CAD build for the part. Positions are in the model's coordinates, mm. A direction names the side the tool comes from. Round coordinates to 2 decimals unless told otherwise and drop trailing zeros. Loops run counter-clockwise (first coordinate to the right, second up) from the corner with the lowest first, then second, coordinate; pieces in that order, holes last.
```python
from build123d import *

# Parameters (mm, degrees)
SKETCH_1_R          = 4
EXTRUDE_1_DEPTH     = 1.5
SKETCH_2_R          = 2.9
EXTRUDE_2_DEPTH     = 5
CUT_EXTRUDE_1_REACH = 10.617
SKETCH_3_R          = 1.6


with BuildPart() as part:
    # 草图1 → 凸台-拉伸1 (new body)
    with BuildSketch(Plane(origin=(0, 0, 0), x_dir=(1, 0, 0), z_dir=(0, 1, 0))):
        with Locations(Location((0, 0, 0), (0, 0, 270))):
            Circle(SKETCH_1_R)
    extrude(amount=EXTRUDE_1_DEPTH)

    # 草图2 → 凸台-拉伸2 (add)
    with BuildSketch(Plane(origin=(0, 1.5, 0), x_dir=(1, 0, 0), z_dir=(0, 1, 0))):
        with Locations(Location((0, 0, 0), (0, 0, 270))):
            Circle(SKETCH_2_R)
    extrude(amount=EXTRUDE_2_DEPTH)

    # 草图3 → 切除-拉伸1 (cut, up to next)
    with BuildSketch(Plane(origin=(0, 6.5, 0), x_dir=(1, 0, 0), z_dir=(0, 1, 0)), mode=Mode.PRIVATE) as cut_extrude_1_sk1:
        with Locations(Location((0, 0, 0), (0, 0, 270))):
            Circle(SKETCH_3_R)
    cut_extrude_1_tool1 = extrude(cut_extrude_1_sk1.sketch, amount=-CUT_EXTRUDE_1_REACH, mode=Mode.PRIVATE) & part.part
    add(cut_extrude_1_tool1.solids().sort_by_distance((0, 6.5, 0))[0], mode=Mode.SUBTRACT)


solid = part.part
```
Item 1: Cut at A-A, the plane x = 0. Give the cut face in (y, z).
Answers follow:
outline: (0, -4) - (1.5, -4) - (1.5, -2.9) - (6.5, -2.9) - (6.5, -1.6) - (0, -1.6) - close; (0, 1.6) - (6.5, 1.6) - (6.5, 2.9) - (1.5, 2.9) - (1.5, 4) - (0, 4) - close
Item 2: Flat gauge pins, fed straight in: P1, Ø1.5, axis at x = 0.5, z = -1.5, coming from the -Y side; P2, Ø1, axis at y = 4, z = -2, coming from the -X side. Where does each tip first touch, or does it go through?
Answers follow:
P1: stops at y = 0
P2: stops at x = -2.48
Item 3: Cut at C-C, the plane y = 2.5. Give the cut face in (x, z).
Answers follow:
outline: circle Ø5.8 at (0, 0); hole circle Ø3.2 at (0, 0)
Item 4: 3-axis set-ups, long thin cutter, end or side, ignore diameter. For faces 1 (the flat face through (-1.25, 6.5, 1.25)), 2 (the cylindrical face through (0.1, 4, -2.9)): which of +Z, -Z, +X, -X, +Y, -Y reach the whole face in a straight line?
Answers follow:
face 1: +Z, -Z, +X, -X, +Y
face 2: +Y
Item 5: Cut at B-B, the plane z = 0. Give the cut face in (x, y).
Answers follow:
outline: (-4, 0) - (-1.6, 0) - (-1.6, 6.5) - (-2.9, 6.5) - (-2.9, 1.5) - (-4, 1.5) - close; (1.6, 0) - (4, 0) - (4, 1.5) - (2.9, 1.5) - (2.9, 6.5) - (1.6, 6.5) - close
Item 6: Cut at D-D, the plane x = -1.75. Give the cut face in (y, z).
Answers follow:
outline: (0, -3.6) - (1.5, -3.6) - (1.5, -2.31) - (6.5, -2.31) - (6.5, 2.31) - (1.5, 2.31) - (1.5, 3.6) - (0, 3.6) - close
Item 7: Probe line 1 (X direction, y = 1.75, z = 0); line 2 (Y direction, x = 3.25, z = -0.5); line 3 (X direction, y = 0.75, z = 0.5). List the from-to ranges inside material, lowest first.
Answers follow:
line 1: x = -2.9 to -1.6, 1.6 to 2.9
line 2: y = 0 to 1.5
line 3: x = -3.97 to -1.52, 1.52 to 3.97
Item 8: Two-plate mould, pull along Z, no slides. Class faces 3 (the flat face through (0, 0, 2)), 4 (the cylindrical face through (-0.97, 3.3, -1.27)), 5 (the cylindrical face through (-3.905, 0.74, -0.867)): released by +Z, released by -Z, zero draft, split by the parting line, or undercut.
Answers follow:
face 3: zero draft
face 4: undercut
face 5: split by the parting line
